from build123d import *

# Parameters (mm, degrees)
EXTRUDE_1_DEPTH = 20
FILLET_1_R      = 5
SCALE_1_SCALE   = 0.2


with BuildPart() as part:
    # 草圖1 → 填料-伸長1 (new body)
    with BuildSketch(Plane.XY):
        Polygon((30, 5), (15, 5), (5, 10), (5, 20), (0, 20), (0, 5), (0, 0), (5, 0), (30, 0), align=None)
    extrude(amount=EXTRUDE_1_DEPTH)

    # 圓角1
    fillet_1_edges = [part.edges().sort_by_distance(p)[0] for p in [
        (2.5, 20, 20),
        (2.5, 20, 0),
    ]]
    fillet(fillet_1_edges, radius=FILLET_1_R)


with BuildPart() as part_1:
    # 縮放比例1: scaled about (10.67100901, 5.776025911, 10)
    add(part.part.scale(SCALE_1_SCALE).moved(Location((8.536807208, 4.620820729, 8))))


solid = part_1.part
Verification items for the finished model (mm, model axes). A direction names the side the tool comes from. Give positions to 0.01 mm unless a question says otherwise; leave off trailing zeros. Write each loop counter-clockwise with the first axis right and the second up, starting at its lowest first coordinate (ties: lowest second). Pieces come first, ordered by that corner, then holes.
(1) Cross-section at C-C (y = 5.95). Enter the section's corners in (x, z).
(2) Cross-section at B-B (z = 11.6). Enter the section's corners in (x, y).
(3) Access from +Z, -Z, +X, -X, +Y, -Y to the whole of each face (thin tool, end or side, straight path). Record for faces 1 (the face through (9, 8.621, 10)), 2 (the face through (13, 5.621, 10)).
(4) Gauge pin test, flat ends, axial feed: pin 1 (1.5 mm diameter, centred on x = 12.5, z = 9.5, fed in from +Y); pin 2 (2 mm diameter, centred on x = 13.5, y = 7.5, fed in from +Z); pin 3 (1 mm diameter, centred on y = 8, z = 10.5, fed in from +X). Record the tip position at first contact, or that the pin passes through.
(5) Cross-section at A-A (x = 9.35). Enter the section's corners in (y, z).
(6) Material ranges on line 1 (X direction, y = 7.9, z = 8.6); line 2 (Y direction, x = 14.2, z = 10.5); line 3 (Y direction, x = 9.4, z = 8.95), recorded low to high.
(7) Cross-section at D-D (z = 9.25). Enter the section's corners in (x, y), plus the area to 3 significant figures.
Worked out:
1. outline: (8.54, 8) - (10.88, 8) - (10.88, 12) - (8.54, 12) - close
2. outline: (8.54, 4.62) - (14.54, 4.62) - (14.54, 5.62) - (11.54, 5.62) - (9.54, 6.62) - (9.54, 8.42) - (8.54, 8.42) - close
3. face 1: +Z, -Z, +X, -X, +Y
3. face 2: +Z, -Z, +X, +Y
4. pin 1: stops at y = 5.62
4. pin 2: passes through
4. pin 3: stops at x = 9.54
5. outline: (4.62, 8) - (7.62, 8) arc R1 ccw to (8.62, 9) - (8.62, 11) arc R1 ccw to (7.62, 12) - (4.62, 12) - close
6. line 1: x = 8.54 to 9.54
6. line 2: y = 4.62 to 5.62
6. line 3: y = 4.62 to 8.62
7. outline: (8.54, 4.62) - (14.54, 4.62) - (14.54, 5.62) - (11.54, 5.62) - (9.54, 6.62) - (9.54, 8.62) - (8.54, 8.62) - close
7. area: 10.0 mm2
